```python
from build123d import *

# Parameters (mm, degrees)
SKETCH1_R           = 6
BOSS_EXTRUDE1_DEPTH = 1.5875
EXTRUDE_THIN1_DEPTH = 25.4
CIRPATTERN1_COUNT   = 4
MIRROR1_DEPTH       = 25.4
MIRROR1_2_OUTLINE_R = 6
MIRROR1_2_DEPTH     = 1.5875


# Read off the part's stored shape, not the designer's step: Mirror1
with BuildPart() as part:
    # Sketch1 → Boss-Extrude1 (new body)
    with BuildSketch(Plane(origin=(0, 0, 0), x_dir=(1, 0, 0), z_dir=(0, 1, 0))):
        Polygon((-22.225, 0), (-15.875, 6.35), (15.875, 6.35), (22.225, 0), (15.875, -6.35), (-15.875, -6.35), align=None)
        with Locations(Location((-9.525, 0, 0), (0, 0, 270))):
            Circle(SKETCH1_R, mode=Mode.SUBTRACT)
        with Locations(Location((9.525, 0, 0), (0, 0, 270))):
            Circle(SKETCH1_R, mode=Mode.SUBTRACT)
    boss_extrude1 = extrude(amount=BOSS_EXTRUDE1_DEPTH)

    # Sketch2 → Extrude-Thin1 (add)
    with BuildSketch(Plane(origin=(0, 0, 0), x_dir=(1, 0, 0), z_dir=(0, 1, 0))):
        Polygon((-23.347532015, 0), (-16.203782015, -7.14375), (16.203782015, -7.14375), (23.347532015, 0), (16.203782015, 7.14375), (-16.203782015, 7.14375), align=None)
        Polygon((-22.225, 0), (-15.875, -6.35), (15.875, -6.35), (22.225, 0), (15.875, 6.35), (-15.875, 6.35), align=None, mode=Mode.SUBTRACT)
    extrude_thin1 = extrude(amount=EXTRUDE_THIN1_DEPTH)

    # CirPattern1: Boss-Extrude1, Extrude-Thin1 ×4 about axis
    cirpattern1_axis = Axis((0, 0, -22.786266008), (0, 1, 0))
    add([boss_extrude1.rotate(cirpattern1_axis, i * 360 / CIRPATTERN1_COUNT) for i in range(1, CIRPATTERN1_COUNT)])
    add([extrude_thin1.rotate(cirpattern1_axis, i * 360 / CIRPATTERN1_COUNT) for i in range(1, CIRPATTERN1_COUNT)])

    # Mirror1 outline → Mirror1 (add)
    with BuildSketch(Plane(origin=(0, 0, 0), x_dir=(1, 0, 0), z_dir=(0, 1, 0))):
        Polygon((-16.436266008, -38.661266008), (-22.786266008, -45.011266008), (-29.136266008, -38.661266008), (-29.136266008, -6.911266008), (-22.786266008, -0.561266008), (-23.347532015, 0), (-29.930016008, -6.582483992), (-29.930016008, -38.990048023), (-16.203782015, -52.716282015), (16.203782015, -52.716282015), (29.930016008, -38.990048023), (29.930016008, -6.582483992), (23.347532015, 0), (22.786266008, -0.561266008), (29.136266008, -6.911266008), (29.136266008, -38.661266008), (22.786266008, -45.011266008), (16.436266008, -38.661266008), (16.436266008, -6.911266008), (16.203782015, -7.14375), (15.642516008, -7.14375), (15.642516008, -38.428782015), (-15.642516008, -38.428782015), (-15.642516008, -7.14375), (-16.203782015, -7.14375), (-16.436266008, -6.911266008), align=None)
        Polygon((15.875, -39.222532015), (22.225, -45.572532015), (15.875, -51.922532015), (-15.875, -51.922532015), (-22.225, -45.572532015), (-15.875, -39.222532015), align=None, mode=Mode.SUBTRACT)
    extrude(amount=MIRROR1_DEPTH)

    # Mirror1 2 outline → Mirror1 2 (add)
    # profile 1 of 3: a face of its own
    with BuildSketch(Plane(origin=(0, 0, 0), x_dir=(1, 0, 0), z_dir=(0, 1, 0))):
        Polygon((15.875, -51.922532015), (22.225, -45.572532015), (15.875, -39.222532015), (-15.875, -39.222532015), (-22.225, -45.572532015), (-15.875, -51.922532015), align=None)
        with Locations((-9.525, -45.572532015)):
            Circle(MIRROR1_2_OUTLINE_R, mode=Mode.SUBTRACT)
        with Locations((9.525, -45.572532015)):
            Circle(MIRROR1_2_OUTLINE_R, mode=Mode.SUBTRACT)
    # profile 2 of 3: a face of its own
    with BuildSketch(Plane(origin=(0, 0, 0), x_dir=(1, 0, 0), z_dir=(0, 1, 0))):
        Polygon((-29.136266008, -38.661266008), (-22.786266008, -45.011266008), (-16.436266008, -38.661266008), (-16.436266008, -6.911266008), (-22.786266008, -0.561266008), (-29.136266008, -6.911266008), align=None)
        with Locations((-22.786266008, -32.311266008)):
            Circle(MIRROR1_2_OUTLINE_R, mode=Mode.SUBTRACT)
        with Locations((-22.786266008, -13.261266008)):
            Circle(MIRROR1_2_OUTLINE_R, mode=Mode.SUBTRACT)
    # profile 3 of 3: a face of its own
    with BuildSketch(Plane(origin=(0, 0, 0), x_dir=(1, 0, 0), z_dir=(0, 1, 0))):
        Polygon((22.786266008, -0.561266008), (16.436266008, -6.911266008), (16.436266008, -38.661266008), (22.786266008, -45.011266008), (29.136266008, -38.661266008), (29.136266008, -6.911266008), align=None)
        with Locations((22.786266008, -32.311266008)):
            Circle(MIRROR1_2_OUTLINE_R, mode=Mode.SUBTRACT)
        with Locations((22.786266008, -13.261266008)):
            Circle(MIRROR1_2_OUTLINE_R, mode=Mode.SUBTRACT)
    extrude(amount=MIRROR1_2_DEPTH)


solid = part.part
```
Build history of the part. All positions in model axes, mm. A direction names the side the tool comes from. Give positions to 0.01 mm unless a question says otherwise; leave off trailing zeros. Loops run counter-clockwise (first coordinate to the right, second up) from the corner with the lowest first, then second, coordinate; pieces in that order, holes last. Notation, with made-up numbers: (55, -3) - (82, -3) arc R35 ccw to (82, 29) - close; hole circle Ø7 at (75.25, 81). An arc over 180 degrees is marked (long way). Use a Markdown table: item, result.
(1) Wall check: line 1 along Z through (x, y) = (-7.5, 11); line 2 along X through (y, z) = (0.85, 0) (3 decimals); line 3 along X through (y, z) = (9.25, -38.5). Give the ranges that are in metal, low to high.
Taken from the geometry:
| item | result |
|---|---|
| line 1 | -52.72 to -51.92, -39.22 to -38.43, -7.14 to -6.35, 6.35 to 7.14, 38.43 to 39.22, 51.92 to 52.72 |
| line 2 | -23.348 to -15.525, -3.525 to 3.525, 15.525 to 23.348 |
| line 3 | -29.93 to -29.14, -16.44 to 16.44, 29.14 to 29.93 |
(2) Band-saw the part on C-C (x = -25). Give the number of separate pieces and of enclosed holes in the cut face, and give its area (3 significant figures).
Taken from the geometry:
| item | result |
|---|---|
| separate pieces | 6 |
| enclosed holes | 0 |
| area | 170 mm2 |
(3) Drop flat-ended pins along their axis: pin 1 Ø6.5 at (x, z) = (21.5, 22.5) entering from +Y; pin 2 Ø8 at (x, y) = (-20.5, 8.5) entering from -Z; pin 3 Ø4 at (y, z) = (4.5, -0.5) entering from -X. Give the stop position or say it passes through.
Taken from the geometry:
| item | result |
|---|---|
| pin 1 | y = 1.59 |
| pin 2 | z = -52.42 |
| pin 3 | x = -25.85 |
(4) Band-saw the part on A-A (x = -1). Give the cut face in (y, z).
Taken from the geometry:
| item | result |
|---|---|
| outline | (0, -52.72) - (25.4, -52.72) - (25.4, -51.92) - (1.59, -51.92) - (1.59, -39.22) - (25.4, -39.22) - (25.4, -38.43) - (0, -38.43) - close; (0, -7.14) - (25.4, -7.14) - (25.4, -6.35) - (1.59, -6.35) - (1.59, 6.35) - (25.4, 6.35) - (25.4, 7.14) - (0, 7.14) - close; (0, 38.43) - (25.4, 38.43) - (25.4, 39.22) - (1.59, 39.22) - (1.59, 51.92) - (25.4, 51.92) - (25.4, 52.72) - (0, 52.72) - close |
(5) Which spindle directions (+Z, -Z, +X, -X, +Y, -Y) get a long thin tool onto all of the face, cutting with end or side? Do faces 1 (the face through (29.136, 13, 23)), 2 (the face through (15.643, 13, 23)), 3 (the face through (29.93, 13, 23)). Say none if no direction does.
Taken from the geometry:
| item | result |
|---|---|
| face 1 | +Y |
| face 2 | +Y, -Y |
| face 3 | +Z, -Z, +X, +Y, -Y |
(6) Pull direction X, two halves, no side cores. Call faces 4 (the face through (-15.382, 0.783, -1.301)), 5 (the face through (-29.93, 13, 23)), 6 (the face through (22.97, 12.52, 45.95)): +X half, -X half, draft (parallel to the pull), parting line (faces both ways), or undercut.
Taken from the geometry:
| item | result |
|---|---|
| face 4 | undercut |
| face 5 | -X half |
| face 6 | +X half |
(7) Band-saw the part on B-B (z = -34). Give the cut face in (x, y), and give its area (3 significant figures).
Taken from the geometry:
| item | result |
|---|---|
| outline | (-29.93, 0) - (-28.54, 0) - (-28.54, 1.59) - (-29.14, 1.59) - (-29.14, 25.4) - (-29.93, 25.4) - close; (-17.03, 0) - (-15.64, 0) - (-15.64, 25.4) - (-16.44, 25.4) - (-16.44, 1.59) - (-17.03, 1.59) - close; (15.64, 0) - (17.03, 0) - (17.03, 1.59) - (16.44, 1.59) - (16.44, 25.4) - (15.64, 25.4) - close; (28.54, 0) - (29.93, 0) - (29.93, 25.4) - (29.14, 25.4) - (29.14, 1.59) - (28.54, 1.59) - close |
| area | 84.4 mm2 |
